The listing builds one solid part. Answer for the finished solid, in the listing's coordinates (mm). Face numbers are marked on the shaded views. A direction names the side the tool comes from. Round coordinates to 2 decimals unless told otherwise and drop trailing zeros. Order: outer loops, then holes, each group sorted by start corner. A loop starts at its lowest first (then second) coordinate and runs counter-clockwise, first axis right, second up. Notation, with made-up numbers: (-13.75, 36) -> (23.25, 36) arc R14 ccw to (23.25, 56) -> close; hole circle Ø10 at (9, 5.5). An arc over 180 degrees is marked (long way). Answer in a Markdown table with one row per item. Add a question column.
```python
from build123d import *

# Parameters (mm, degrees)
BASE_FLANGE1_DEPTH    = 112.5
SKETCH4_R             = 2.75
CUT_EXTRUDE1_DEPTH    = 10
SKETCH5_W             = 145
SKETCH5_H             = 10
CUT_EXTRUDE2_DEPTH    = 70
CHAMFER1_SIZE         = 2
M5_TAPPED_HOLE1_D     = 4.2
M5_TAPPED_HOLE1_DEPTH = 12.4
M5_TAPPED_HOLE1_TIP   = 1.2618073


# Sheet-metal steps are written as plain solids
with BuildPart() as part:
    # Sketch1 → Base-Flange1 (new, symmetric)
    with BuildSketch(Plane.XY):
        with BuildLine():
            Line((0, 30), (0, 6))
            ThreePointArc((0, 6), (-1.757359313, 1.757359313), (-6, 0))
            Line((-6, 0), (-22, 0))
            Line((-22, 0), (-22, 3))
            Line((-22, 3), (-6, 3))
            ThreePointArc((-6, 3), (-3.878679656, 3.878679656), (-3, 6))
            Line((-3, 6), (-3, 30))
            Line((-3, 30), (0, 30))
        make_face()
    extrude(amount=BASE_FLANGE1_DEPTH, both=True)

    # Sketch4 → Cut-Extrude1 (cut)
    with BuildSketch(Plane(origin=(0, 3, 0), x_dir=(1, 0, 0), z_dir=(0, 1, 0))):
        with Locations(Location((-14, -90, 0), (0, 0, 180))):
            Circle(SKETCH4_R)
        with Locations((-14, 90)):
            Circle(SKETCH4_R)
    extrude(amount=-CUT_EXTRUDE1_DEPTH, mode=Mode.SUBTRACT)

    # Sketch5 → Cut-Extrude2 (cut)
    with BuildSketch(Plane(origin=(0, 0, 0), x_dir=(0, 0, -1), z_dir=(1, 0, 0))):
        with Locations((0, 5)):
            Rectangle(SKETCH5_W, SKETCH5_H)
    extrude(amount=-CUT_EXTRUDE2_DEPTH, mode=Mode.SUBTRACT)

    # Chamfer1
    chamfer1_edges = [part.edges().sort_by_distance(p)[0] for p in [
        (-1.5, 30, 112.5),
        (-22, 1.5, 72.5),
        (-22, 1.5, -72.5),
        (-22, 1.5, 112.5),
        (-1.5, 30, -112.5),
        (-22, 1.5, -112.5),
    ]]
    chamfer(chamfer1_edges, length=CHAMFER1_SIZE)

    # M5 Tapped Hole1
    with Locations(Plane(origin=(0, 18, 90), x_dir=(0, 0, 1), z_dir=(1, 0, 0))):
        with Locations((0, 0), (-180, 0)):
            Hole(M5_TAPPED_HOLE1_D / 2, depth=M5_TAPPED_HOLE1_DEPTH)
            with Locations((0, 0, -(M5_TAPPED_HOLE1_DEPTH + M5_TAPPED_HOLE1_TIP / 2))):  # 118° drill point
                Cone(0, M5_TAPPED_HOLE1_D / 2, M5_TAPPED_HOLE1_TIP, mode=Mode.SUBTRACT)


solid = part.part
```
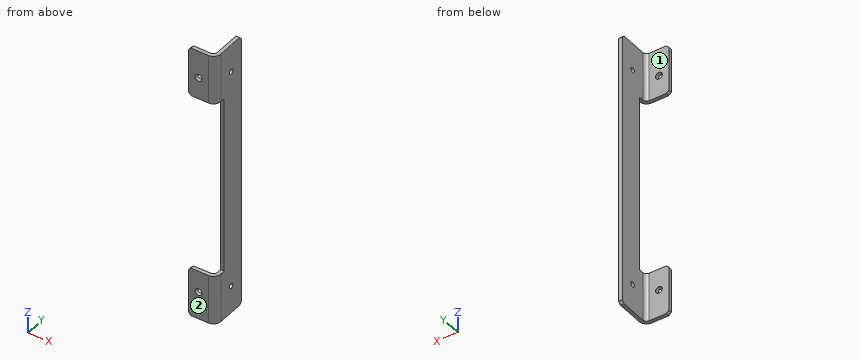
Item 1: The part is cut by section D-D, the plane z = -36. Give the vertices of the cut face in (x, y).
Item 2: The part is cut by section C-C, the plane y = 18. Give the vertices of the cut face in (x, z).
Item 3: Flat-ended cylindrical pins translate along their axes: P1, Ø3, axis at y = 10, z = 34, coming from the -X side; P2, Ø2.5, axis at y = 18, z = -90, coming from the +X side; P3, Ø8, axis at x = -12, z = -86.5, coming from the +Y side; P4, Ø2.5, axis at x = -2, z = -2, coming from the -Y side. Find the tip coordinate at first contact, or state that the pin passes through.
Item 4: The part is cut by section A-A, the plane x = -14. Give the vertices of the cut face in (y, z), and give its area (3 significant figures).
Item 5: A tool of negligible diameter and unlimited length cuts with its end or side. For the marked faces 1 and 2, from which of +Z, -Z, +X, -X, +Y, -Y can it reach the whole face along a straight path? Write none if from no direction.
Item 6: Find the intervals of material crossed by probe 1 along Z at (x, y) = (-0.95, 18); probe 2 along Z at (x, y) = (-14, 0.75); probe 3 along X at (y, z) = (17.25, 34), in increasing order. Write a range as [from, to].
Item 7: The part is cut by section B-B, the plane z = 90. Give the vertices of the cut face in (x, y), and give its area (3 significant figures).
Resolved:
| question | item | result |
|---|---|---|
| 1 | outline | (-3, 10) -> (0, 10) -> (0, 30) -> (-3, 30) -> close |
| 2 | outline | (-3, -112.5) -> (0, -112.5) -> (0, -92.1) -> (-3, -92.1) -> close; (-3, -87.9) -> (0, -87.9) -> (0, 87.9) -> (-3, 87.9) -> close; (-3, 92.1) -> (0, 92.1) -> (0, 112.5) -> (-3, 112.5) -> close |
| 3 | P1 | x = -3 |
| 3 | P2 | through |
| 3 | P3 | y = 3 |
| 3 | P4 | y = 10 |
| 4 | outline | (0, -112.5) -> (3, -112.5) -> (3, -92.75) -> (0, -92.75) -> close; (0, -87.25) -> (3, -87.25) -> (3, -72.5) -> (0, -72.5) -> close; (0, 72.5) -> (3, 72.5) -> (3, 87.25) -> (0, 87.25) -> close; (0, 92.75) -> (3, 92.75) -> (3, 112.5) -> (0, 112.5) -> close |
| 4 | area | 207 mm2 |
| 5 | face 1 | +Z, -Z, -X, +Y |
| 5 | face 2 | +Z, -Z, +X, -X, -Y |
| 6 | probe 1 | [-112.5, -92.1], [-87.9, 87.9], [92.1, 112.5] |
| 6 | probe 2 | [-112.5, -92.75], [-87.25, -72.5], [72.5, 87.25], [92.75, 112.5] |
| 6 | probe 3 | [-3, 0] |
| 7 | outline | (-22, 0) -> (-16.75, 0) -> (-16.75, 3) -> (-22, 3) -> close; (-11.25, 0) -> (-6, 0) arc R6 ccw to (0, 6) -> (0, 15.9) -> (-3, 15.9) -> (-3, 6) arc R3 cw to (-6, 3) -> (-11.25, 3) -> close; (-3, 20.1) -> (0, 20.1) -> (0, 30) -> (-3, 30) -> close |
| 7 | area | 112 mm2 |
